Can you work these out from the model? Positions are in its coordinate system, mm. Round coordinates to 2 decimals unless told otherwise and drop trailing zeros. Write each loop counter-clockwise with the first axis right and the second up, starting at its lowest first coordinate (ties: lowest second). Pieces come first, ordered by that corner, then holes. Notation, with made-up numbers: M 52.5,25.25 L 58.5,25.25 A11 cw 58.5,46.25 Z; hole C 23.25,13.25 d8. An arc over 180 degrees is marked long. Answer in a Markdown table with one row per item. Add a question column.
(1) Suppose I cut it at A-A, the plane x = 2034. Write out the boundary of the cut face in (y, z), then the cut area to 3 significant figures.
(2) If I drill on probe 1 along Z at (x, y) = (1812.5, 2514); probe 2 along Z at (x, y) = (1710, 2533.5); probe 3 along Z at (x, y) = (2030, 2657.5), over which ranges is the centre line in solid material (lowest first)?
(3) I'm going to push flat-ended pins straight in: pin 1 (2 mm diameter, centred on y = 2566.5, z = -3639.5, fed in from +X); pin 2 (25 mm diameter, centred on y = 2538, z = -3744.5, fed in from -X); pin 3 (12 mm diameter, centred on y = 2661, z = -3807, fed in from +X). Where does each tip first touch, or does it pass through?
(4) Suppose I cut it at C-C, the plane y = 2654. Write out the boundary of the cut face in (x, z), then the cut area to 3 significant figures.
(5) Suppose I cut it at D-D, the plane z = -3612.5. Write out the boundary of the cut face in (x, y), then the cut area to 3 significant figures.
(6) Suppose I cut it at B-B, the plane z = -3774. Write out the boundary of the cut face in (x, y).
Autodesk Inventor part; units mm, degrees
ref_plane "Work Plane2" through (0, 0, -7900) normal (0, 0, 1) x (1, 0, 0)
ref_plane "Work Plane3" through (2500, 0, 0) normal (1, 0, 0) x (0, 1, 0)
ref_plane "Work Plane4" through (1945.737, 1551.2045, -2616.5476) normal (0, -0.9956912, -0.0927309) x (1, 0, 0)
sketch "Sketch1" plane through (0, 0, 0) normal (0, 0, 1) x (1, 0, 0)
  line L0 (2948.6488, 634.5525) -> (2841.4489, 559.4904)
  line L1 (2841.4489, 559.4904) -> (2956.2003, 395.6085)
  line L2 (2956.2003, 395.6085) -> (3063.4001, 470.6706)
  line L3 (1051.1773, 2444.1167) -> (976.8907, 2338.0244)
  line L4 (976.8907, 2338.0244) -> (1140.7211, 2223.3091)
  line L5 (1140.7211, 2223.3091) -> (1215.0077, 2329.4014)
  line L6 (-383.8501, 3232.1868) -> (-383.8501, 3052.6308)
  arc A0 (4065.9398, -2152.4924) -> (-383.8501, 3052.6308) centre (-4485.4868, -4958.3977) ccw
  arc A1 (1051.1773, 2444.1167) -> (-383.8501, 3232.1868) centre (-3980.604, -5017.8654) ccw
  arc A2 (2948.6488, 634.5525) -> (1215.0077, 2329.4014) centre (-4152.392, -4894.9339) ccw
  arc A3 (4300.883, -1939.8955) -> (3063.4001, 470.6706) centre (-4233.2291, -4798.0297) ccw
  arc A4 (4065.9398, -2152.4924) -> (4300.883, -1939.8955) centre (3657.2708, -1464.7499) ccw
  point P0 (0, 0)
  point P1 (4065.924, -2152.4924)
  point P2 (4065.924, -2152.4924)
  dimension "d8" = 9000
  dimension "d9" = 9000
  dimension "d10" = 9000
  dimension "d11" = 9000
  dimension "d12" = 800
ref_plane "Work Plane2" through (0, 0, -7900) normal (0, 0, 1) x (1, 0, 0)
ref_plane "Work Plane1" through (0, 0, 0) normal (0, 0, 1) x (1, 0, 0)
sketch "Sketch2" plane through (0, 0, -7900) normal (0, 0, 1) x (1, 0, 0)
  arc A0 (895.257, 3171.2695) -> (-383.8658, 4018.7524) centre (-4697.1096, -3880.3569) ccw
  line L0 (-383.8658, 4018.7524) -> (-383.8658, 3839.1061)
  arc A1 (4065.924, -2152.4924) -> (-383.8658, 3839.1061) centre (-4733.9746, -4039.7614) ccw
  line L1 (895.257, 3171.2695) -> (830.4728, 3059.0601)
  line L2 (830.4728, 3059.0601) -> (1003.6891, 2959.0536)
  line L3 (1068.4733, 3071.2631) -> (1003.6891, 2959.0536)
  arc A2 (2750.1419, 1279.62) -> (1068.4733, 3071.2631) centre (-4591.4319, -3926.2703) ccw
  line L4 (2750.1419, 1279.62) -> (2643.8882, 1205.2246)
  line L5 (2643.8882, 1205.2246) -> (2759.146, 1041.7698)
  line L6 (2865.5448, 1116.2711) -> (2759.146, 1041.7698)
  arc A3 (4310.9102, -1926.005) -> (2865.5448, 1116.2711) centre (-4397.3898, -4198.7812) ccw
  arc A4 (4065.924, -2152.4924) -> (4310.9102, -1926.005) centre (3657.2831, -1464.7333) ccw
  point P0 (0, 0)
  dimension "d7" = 800
loft "Loft1" add profiles "Sketch1", "Sketch2"
ref_plane "Work Plane3" through (2500, 0, 0) normal (1, 0, 0) x (0, 1, 0)
sketch "Sketch3" plane through (2500, 0, 0) normal (1, 0, 0) x (0, 1, 0)
  line L0 (2569.5835, -3718.0946) -> (1551.2045, -2616.5476)
  line L1 (1551.2045, -2616.5476) -> (1738.7871, -4630.7013)
  line L2 (1738.7871, -4630.7013) -> (2569.5835, -3718.0946)
  line L3 (4228.9662, 279.606) -> (-2269.9695, 279.606)
  line L4 (-2269.9695, 279.606) -> (-2269.9695, -8192.2559)
  line L5 (-2269.9695, -8192.2559) -> (4228.9662, -8192.2559)
  line L6 (4228.9662, -8192.2559) -> (4228.9662, 279.606)
  point P0 (0, 0)
extrude "Extrusion1" cut sketch "Sketch3" along normal through all both and the other way through all
ref_plane "Work Plane4" through (1945.737, 1551.2045, -2616.5476) normal (0, -0.9956912, -0.0927309) x (1, 0, 0)
sketch "Sketch5" plane through (1945.737, 1551.2045, -2616.5476) normal (0, -0.9956912, -0.0927309) x (1, 0, 0)
  line L0 (347.8734, 0) -> (290.3896, -2022.8698)
  point P0 (-1945.737, 2749.1181)
ref_plane "Work Plane5" through (2293.6104, 1551.2045, -2616.5476) normal (-0.6425282, -0.7644369, -0.052856) x (-0.0284055, 0.0926935, -0.9952894)
sketch "Sketch6" plane through (2293.6104, 1551.2045, -2616.5476) normal (-0.6425282, -0.7644369, -0.052856) x (-0.0284055, 0.0926935, -0.9952894)
  line L0 (-1061.9028, -2252.9112) -> (2197.0944, -2252.9112)
  line L1 (2197.0944, -2252.9112) -> (2197.0944, 343.7273)
  line L2 (2197.0944, 343.7273) -> (-1061.9028, 343.7273)
  line L3 (-1061.9028, 343.7273) -> (-1061.9028, -2252.9112)
  point P0 (-2682.8576, -979.2829)
extrude "Extrusion2" cut sketch "Sketch6" against normal through all
ref_plane "Work Plane6" through (2293.6104, 1551.2045, -2616.5476) normal (-0.9995965, -0.0026341, 0.0282831) x (-0.0284055, 0.0926935, -0.9952894)
sketch "Sketch7" plane through (2293.6104, 1551.2045, -2616.5476) normal (-0.6425282, -0.7644369, -0.052856) x (-0.0284055, 0.0926935, -0.9952894)
  line L0 (0, 0) -> (1222.5973, -1418.5767)
  line L1 (1222.5973, -1418.5767) -> (2023.6864, 0)
  point P0 (-2682.8576, -979.2829)
sketch "Sketch8" plane through (2293.6104, 1551.2045, -2616.5476) normal (-0.9995965, -0.0026341, 0.0282831) x (-0.0284055, 0.0926935, -0.9952894)
  line L0 (0, 0) -> (1222.5973, -911.8435)
  spline S0 degree 4 poles (2023.6864, 0) (1891.4174, -0.0605) (1759.1485, -0.1112) (1626.8795, -0.1518) (1361.543, -0.2126) (1228.4756, -0.2325) (1095.4081, -0.2417) (831.8573, -0.2379) (701.374, -0.2253) (570.8907, -0.2017) (330.3055, -0.1374) (220.2037, -0.0999) (110.1018, -0.0542) (0, 0) knots 0 0 0 0 0 0.261442 0.261442 0.261442 0.524462 0.524462 0.524462 0.782374 0.782374 0.782374 1 1 1 1 1
  line L1 (1222.5973, -911.8435) -> (2023.6864, 0)
  point P0 (-2682.8576, 1301.8858)
sketch "Sketch9" plane through (2293.6104, 1551.2045, -2616.5476) normal (-0.9995965, -0.0026341, 0.0282831) x (-0.0284055, 0.0926935, -0.9952894)
  line L0 (1222.5973, -911.8435) -> (0, 0)
  line L1 (2023.6864, 0) -> (1222.5973, -911.8435)
  spline S0 degree 4 poles (0, 0) (253.1862, 0) (506.3724, 0) (759.5586, 0) (1265.4802, 0) (1518.2156, 0) (1770.951, 0) (2023.6864, 0) knots 0 0 0 0 0 0.500446 0.500446 0.500446 1 1 1 1 1
  point P0 (-2682.8576, 1301.8858)
extrude "Extrusion3" add sketch "Sketch9" against normal blind 1
sketch "Sketch10" plane through (2294.61, 1551.2071, -2616.5759) normal (0.9995965, 0.0026341, -0.0282831) x (-0.0284055, 0.0926935, -0.9952894)
  line L0 (1222.5973, 911.8435) -> (2011.6459, 13.7052)
  line L1 (1222.5973, 911.8435) -> (1126.4049, 840.1008)
  line L2 (0, 0) -> (1222.5973, 911.8435)
  line L3 (1222.5973, 911.8435) -> (1301.7983, 821.6925)
  line L4 (1301.7983, 821.6925) -> (1376.9241, 887.6934)
  line L5 (1376.9241, 887.6934) -> (1235.027, 1068.2138)
  line L6 (1126.4049, 840.1008) -> (1066.6193, 920.2612)
  line L7 (1066.6193, 920.2612) -> (1235.027, 1068.2138)
  point P0 (-2682.8576, -1301.8858)
  dimension "d31" = 120
  dimension "d32" = 120
  dimension "d33" = 100
  dimension "d34" = 100
extrude "Extrusion5" add sketch "Sketch10" against normal blind 1100
sketch "Sketch16" plane through (2294.61, 1551.2071, -2616.5759) normal (0.9995965, 0.0026341, -0.0282831) x (-0.0284055, 0.0926935, -0.9952894)
  line L0 (0, 0) -> (1126.4049, 840.1008)
  line L1 (1020.1978, 760.8889) -> (1222.5973, 911.8435)
  line L2 (0, 0) -> (-179.2361, -133.6787)
  line L3 (-179.2361, -133.6787) -> (2478.6059, -144.4888)
  line L4 (2478.6059, -144.4888) -> (2023.6864, 0)
  line L5 (1305.5559, 824.9938) -> (1226.6196, 914.8434)
  line L6 (1222.5973, 911.8435) -> (1226.6196, 914.8434)
  point P0 (-2682.8576, -1301.8858)
extrude "Extrusion6" cut sketch "Sketch8" along normal blind 2000
sketch "Sketch17" plane through (2256.6322, 2490.0248, -3836.0174) normal (0.0213399, -0.7268016, 0.6865159) x (0.9995965, 0.0026341, -0.0282831)
  line L0 (0, 0) -> (-979.255, 0)
  line L1 (-1518.239, 0) -> (548.3239, 0)
  line L2 (548.3239, 0) -> (548.3239, -1298.4887)
  line L3 (548.3239, -1298.4887) -> (-1518.239, -1298.4887)
  line L4 (-1518.239, -1298.4887) -> (-1518.239, 0)
  point P0 (-2370.775, 1034.5522)
  point P1 (-1213.4732, 0)
  point P2 (-1999, 0)
extrude "Extrusion7" cut sketch "Sketch17" along normal mid plane 5000
sketch "Sketch18" plane through (2294.61, 1551.2071, -2616.5759) normal (0.9995965, 0.0026341, -0.0282831) x (-0.0284055, 0.0926935, -0.9952894)
  line L0 (1126.4049, 840.1008) -> (1222.5973, 911.8435)
  line L1 (1301.7983, 821.6925) -> (366.6688, 0.1458)
  spline S0 degree 4 poles (366.6688, 0.1458) (275.0016, 0.1179) (183.3344, 0.0844) (91.6672, 0.0451) (0, 0) knots 0 0 0 0 0 1 1 1 1 1
  line L2 (0, 0) -> (1126.4049, 840.1008)
  line L3 (1126.4049, 840.1008) -> (1222.5973, 911.8435)
  line L4 (1222.5973, 911.8435) -> (1301.7983, 821.6925)
  point P0 (-2682.8576, -1301.8858)
  point P1 (1126.4049, 840.1008)
extrude "Extrusion8" cut sketch "Sketch18" along normal mid plane 5000
sketch "Sketch19" plane through (1945.737, 1551.2045, -2616.5476) normal (0, -0.9956912, -0.0927309) x (1, 0, 0)
  line L0 (407.6375, 227.4777) -> (-99.9449, 227.4777)
  line L1 (-99.9449, 227.4777) -> (-99.9449, -459.2513)
  line L2 (-99.9449, -459.2513) -> (407.6375, -459.2513)
  line L3 (407.6375, -459.2513) -> (407.6375, 227.4777)
  point P0 (-1945.737, 2749.1181)
extrude "Extrusion9" cut sketch "Sketch19" along normal mid plane 100
sketch "Sketch20" plane through (929.9316, 2569.5835, -3718.0946) normal (0, 0.7394745, -0.6731846) x (1, 0, 0)
  line L0 (3.9942, -0.4392) -> (230.3898, -0.0226)
  line L1 (-207.8079, -0.0226) -> (-207.8079, 338.0495)
  line L2 (-207.8079, 338.0495) -> (230.3898, 338.0495)
  line L3 (230.3898, 338.0495) -> (230.3898, -0.0226)
  line L4 (-207.8079, -0.0226) -> (-207.8079, -237.6599)
  line L5 (-207.8079, -237.6599) -> (230.3898, -237.6599)
  line L6 (230.3898, -237.6599) -> (230.3898, 129.1543)
  point P0 (-929.9316, -1019.6322)
extrude "Extrusion10" cut sketch "Sketch20" against normal blind 1100
properties part number "panel_block_02" material "Wood (Maple)"
Calculated:
| question | item | result |
|---|---|---|
| 1 | outline | M 2489.44,-3829.72 L 2562.12,-3898.43 L 2728.7,-3740.35 L 2565.76,-3586.32 L 2491.5,-3653.3 L 2571.85,-3742.47 Z |
| 1 | area | 36,500 mm² |
| 2 | probe 1 | -3847.22 to -3796.83, -3672.65 to -3626.21 |
| 2 | probe 2 | -3863.01 to -3773, -3691.69 to -3605.48 |
| 2 | probe 3 | -3807.8 to -3672.93 |
| 3 | pin 1 | x = 2263.02 |
| 3 | pin 2 | x = 1159.3 |
| 3 | pin 3 | x = 2258.17 |
| 4 | outline | M 1158.22,-3784.27 L 2257.71,-3818.13 L 2261.74,-3675.61 L 1162.1,-3647.23 Z |
| 4 | area | 154,000 mm² |
| 5 | outline | M 1163.18,2617.23 L 1163.47,2507.13 L 2263.81,2544.55 L 2263.7,2587.19 Z |
| 5 | area | 84,000 mm² |
| 6 | outline | M 1158.48,2664.83 L 1158.87,2518.69 L 1160.32,2518.69 L 1160.32,2516.42 L 2259.23,2548.68 L 2258.83,2700.54 Z |
